Autodesk Inventor part; units mm, degrees
ref_plane "YZ Plane" through (0, 0, 0) normal (1, 0, 0) x (0, 1, 0)
ref_plane "XZ Plane" through (0, 0, 0) normal (0, 1, 0) x (-1, 0, 0)
ref_plane "XY Plane" through (0, 0, 0) normal (0, 0, 1) x (1, 0, 0)
sketch "Sketch3" plane through (0, 0, 0) normal (0, 0, 1) x (1, 0, 0)
  line L0 (0, 0) -> (60, 0)
  line L1 (60, 0) -> (60, 12)
  line L2 (60, 12) -> (0, 12)
  line L3 (0, 12) -> (0, 0)
  circle A0 centre (40, 4.5) radius 1.5
  circle A1 centre (5, 6) radius 1.5
  dimension "d0" = 60
  dimension "d2" = 3
  dimension "d3" = 4.5
  dimension "d4" = 12
  dimension "d8" = 20
  dimension "d17" = 3
  dimension "d18" = 5
extrude "Extrusion1" add sketch "Sketch3" along normal blind 3
sketch "Sketch4" plane through (0, 0, 3) normal (0, 0, 1) x (1, 0, 0)
  line L0 (60, 12) -> (0, 12)
  line L1 (45.9, 0) -> (51.9, 0)
  line L2 (51.9, 0) -> (51.9, 12)
  line L3 (51.9, 12) -> (45.9, 12)
  line L4 (45.9, 12) -> (45.9, 0)
  circle A0 centre (40, 4.5) radius 1.5
  point P0 (0, 0)
  dimension "d9" = 6
  dimension "d10" = 5.9
extrude "Extrusion2" add sketch "Sketch4" against normal blind 35 contours L2 L1 L4 L0
sketch "Sketch5" plane through (51.9, 0, 0) normal (1, 0, 0) x (0, 0, -1)
  line L0 (32, 0) -> (32, 12) construction
  line L1 (0, 6) -> (0, 3) construction
  line L2 (32, 6) -> (0, 6) construction
  circle A0 centre (27, 6) radius 1.5
  point P0 (0, 0)
  dimension "d13" = 3
  dimension "d14" = 5
extrude "Extrusion3" cut sketch "Sketch5" against normal through all
properties part number "thumper-bumper-solenoid-interface"
Here's how the part is built. I have some questions about the finished solid (model axes, mm). A direction names the side the tool comes from. Round coordinates to 2 decimals unless told otherwise and drop trailing zeros. Order: outer loops, then holes, each group sorted by start corner. A loop starts at its lowest first (then second) coordinate and runs counter-clockwise, first axis right, second up. Notation, with made-up numbers: M 21,-4 L 62,-4 A16 cw 62,5 Z; hole C -9.5,23.5 d10. An arc over 180 degrees is marked long. One line per question, with ' | ' between items.
1) Imagine slicing it at A-A, the plane z = -27. Write out the boundary of the cut face in (x, y).
Checked values:
outline: M 45.9,0 L 51.9,0 L 51.9,4.5 L 45.9,4.5 Z; M 45.9,7.5 L 51.9,7.5 L 51.9,12 L 45.9,12 Z
2) On a 3-axis mill with a long thin cutter (end or side, diameter ignored), from which of +Z, -Z, +X, -X, +Y, -Y can I reach the whole of each face in a straight line? I mean faces 4 (the flat face through (51.9, 6, -16)), 5 (the flat face through (45.9, 6, -16)), 6 (the flat face through (49, 6, -32)). Say none if no direction works.
Checked values:
face 4: -Z, +X, +Y, -Y | face 5: -Z, -X, +Y, -Y | face 6: -Z, +X, -X, +Y, -Y
3) Imagine slicing it at B-B, the plane y = 11.25. Write out the boundary of the cut face in (x, z), plus the area to 3 significant figures.
Checked values:
outline: M 0,0 L 45.9,0 L 45.9,-32 L 51.9,-32 L 51.9,0 L 60,0 L 60,3 L 0,3 Z | area: 372 mm²
4) We'd pull the mould along Z, two halves only. Please class faces 1 (the cylindrical face through (48.94, 6.07, -25.5)), 2 (the flat face through (39, 12, 1)), 3 (the flat face through (23, 6, 0)): released by +Z, released by -Z, zero draft, split by the parting line, or undercut.
Checked values:
face 1: undercut | face 2: zero draft | face 3: released by -Z
5) I need wall thicknesses on line 1 (Y direction, x = 40, z = 1.3); line 2 (Y direction, x = 50.35, z = -27); line 3 (X direction, y = 1.5, z = -17). Which ranges of each line are inside material? Lowest first, please.
Checked values:
line 1: y = 0 to 3, 6 to 12 | line 2: y = 0 to 4.5, 7.5 to 12 | line 3: x = 45.9 to 51.9
6) I'm going to push flat-ended pins straight in: pin 1 Ø2 at (y, z) = (9, -20.5) entering from -X; pin 2 Ø3.5 at (y, z) = (4, -15.5) entering from +X. Where does each tip first touch, or does it pass through?
Checked values:
pin 1: stops at x = 45.9 | pin 2: stops at x = 51.9
7) Imagine slicing it at D-D, the plane x = 47.5. Write out the boundary of the cut face in (y, z).
Checked values:
outline: M 0,-32 L 12,-32 L 12,3 L 0,3 Z; hole C 6,-27 d3
8) Imagine slicing it at C-C, the plane x = 5. Write out the boundary of the cut face in (y, z), plus the area to 3 significant figures.
Checked values:
outline: M 0,0 L 4.5,0 L 4.5,3 L 0,3 Z; M 7.5,0 L 12,0 L 12,3 L 7.5,3 Z | area: 27.0 mm²
